Input: part model. Units: mm. Frame: model coordinates. Round coordinates to 2 decimals unless told otherwise and drop trailing zeros. Loops run counter-clockwise (first coordinate to the right, second up) from the corner with the lowest first, then second, coordinate; pieces in that order, holes last.
(1) Cut plane B-B, the plane x = -19. Output: boundary loops of the cut face in (y, z), and give its area (3 significant figures).
(2) Cut plane C-C, the plane z = 0.95. Output: boundary loops of the cut face in (x, y), and give its area (3 significant figures).
(3) Line query: line 1 (X direction, y = 0, z = 1.1); line 2 (Y direction, x = -19, z = 0.75); line 3 (X direction, y = -1, z = 0.55). Output: solid intervals per line, ascending.
(4) First-contact query: pin 1 Ø3 at (x, y) = (-57, 0) entering from +Z. Flat tip, straight axial feed; report the tip coordinate or a pass-through.
(5) Cut plane A-A, the plane y = 0. Output: boundary loops of the cut face in (x, z), and give its area (4 significant figures).
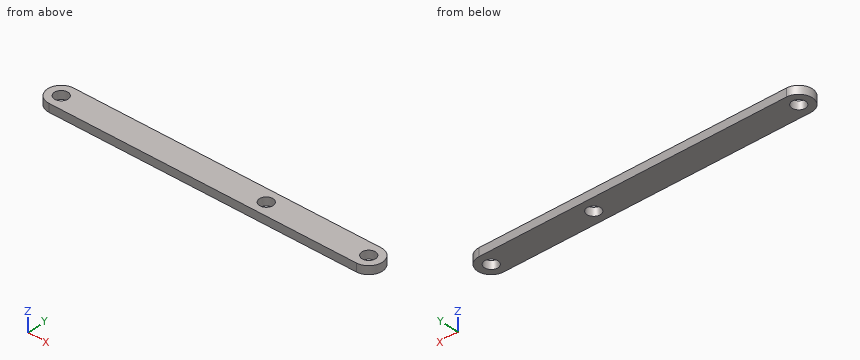
Autodesk Inventor part; units mm, degrees
ref_plane "YZ Plane" through (0, 0, 0) normal (1, 0, 0) x (0, 1, 0)
ref_plane "XZ Plane" through (0, 0, 0) normal (0, 1, 0) x (-1, 0, 0)
ref_plane "XY Plane" through (0, 0, 0) normal (0, 0, 1) x (1, 0, 0)
sketch "Sketch1" plane through (0, 0, 0) normal (0, 0, 1) x (1, 0, 0)
  arc A0 (0, -2.5) -> (0, 2.5) centre (0, 0) ccw
  arc A1 (-57, 2.5) -> (-57, -2.5) centre (-57, 0) ccw
  line L0 (-57, 2.5) -> (0, 2.5)
  line L1 (0, -2.5) -> (-57, -2.5)
  dimension "d0" = 2.5
  dimension "d1" = 2.5
  dimension "d2" = 57
extrude "Extrusion1" add sketch "Sketch1" along normal blind 1.5
sketch "Sketch2" plane through (0, 0, 1.5) normal (0, 0, 1) x (1, 0, 0)
  arc A0 (0, -2.5) -> (0, 2.5) centre (0, 0) ccw
  arc A1 (-57, 2.5) -> (-57, -2.5) centre (-57, 0) ccw
  point P0 (-19, 0)
  dimension "d5" = 38
  dimension "d6" = 19
hole "Hole1" at (-57, 0, 1.5) at (-19, 0, 1.5) at (0, 0, 1.5) direction (0, 0, -1) diameter 2.5 end through all
properties part number "31 - Lever" material "Steel AISI 1020 108 ANLD"
Reported:
1. outline: (-2.5, 0) - (-1.25, 0) - (-1.25, 1.5) - (-2.5, 1.5) - close; (1.25, 0) - (2.5, 0) - (2.5, 1.5) - (1.25, 1.5) - close
1. area: 3.75 mm2
2. outline: (-57, -2.5) - (0, -2.5) arc R2.5 ccw to (0, 2.5) - (-57, 2.5) arc R2.5 ccw to start; hole circle Ø2.5 at (-57, 0); hole circle Ø2.5 at (-19, 0); hole circle Ø2.5 at (0, 0)
2. area: 290 mm2
3. line 1: x = -59.5 to -58.25, -55.75 to -20.25, -17.75 to -1.25, 1.25 to 2.5
3. line 2: y = -2.5 to -1.25, 1.25 to 2.5
3. line 3: x = -59.29 to -57.75, -56.25 to -19.75, -18.25 to -0.75, 0.75 to 2.29
4. pin 1: stops at z = 1.5
5. outline: (-59.5, 0) - (-58.25, 0) - (-58.25, 1.5) - (-59.5, 1.5) - close; (-55.75, 0) - (-20.25, 0) - (-20.25, 1.5) - (-55.75, 1.5) - close; (-17.75, 0) - (-1.25, 0) - (-1.25, 1.5) - (-17.75, 1.5) - close; (1.25, 0) - (2.5, 0) - (2.5, 1.5) - (1.25, 1.5) - close
5. area: 81.75 mm2
